```python
from build123d import *

# Parameters (mm, degrees)
EXTRUDE_THIN2_OUTLINE_R   = 5.5
EXTRUDE_THIN2_OUTLINE_R_2 = 3.5
EXTRUDE_THIN2_DEPTH       = 45
EXTRUDE_THIN2_2_OUTLINE_R = 3.5
EXTRUDE_THIN2_2_DEPTH     = 2
EXTRUDE_THIN2_START       = 43
EXTRUDE_THIN2_3_OUTLINE_R = 3.5
EXTRUDE_THIN2_3_DEPTH     = 2
EXTRUDE_THIN2_4_DEPTH     = 45
EXTRUDE_THIN2_5_DEPTH     = 45
EXTRUDE_THIN2_6_DEPTH     = 45
EXTRUDE_THIN2_7_DEPTH     = 45
EXTRUDE_THIN2_8_OUTLINE_W = 2
EXTRUDE_THIN2_8_OUTLINE_H = 52
EXTRUDE_THIN2_8_DEPTH     = 45
SKETCH4_R                 = 5.5
BOSS_EXTRUDE2_DEPTH       = 0.001
SKETCH6_R                 = 6.759527971
BOSS_EXTRUDE3_DEPTH       = 1
SCALE1_SCALE              = 1.5


# Read off the part's stored shape, not the designer's step: Extrude-Thin2
with BuildPart() as part:
    # Extrude-Thin2 outline → Extrude-Thin2 (new body)
    with BuildSketch(Plane(origin=(0, 0, 0), x_dir=(1, 0, 0), z_dir=(0, 1, 0))):
        Circle(EXTRUDE_THIN2_OUTLINE_R)
        Circle(EXTRUDE_THIN2_OUTLINE_R_2, mode=Mode.SUBTRACT)
    extrude(amount=EXTRUDE_THIN2_DEPTH)

    # Extrude-Thin2 2 outline → Extrude-Thin2 2 (add)
    with BuildSketch(Plane(origin=(0, 0, 0), x_dir=(1, 0, 0), z_dir=(0, 1, 0))):
        Circle(EXTRUDE_THIN2_2_OUTLINE_R)
    extrude(amount=EXTRUDE_THIN2_2_DEPTH)

    # Extrude-Thin2 3 outline → Extrude-Thin2 3 (add)
    with BuildSketch(Plane(origin=(0, 0, 0), x_dir=(1, 0, 0), z_dir=(0, 1, 0)).offset(EXTRUDE_THIN2_START)):
        Circle(EXTRUDE_THIN2_3_OUTLINE_R)
    extrude(amount=EXTRUDE_THIN2_3_DEPTH)



with BuildPart() as body_2:
    # Extrude-Thin2 4 outline → Extrude-Thin2 4 (new body)
    with BuildSketch(Plane(origin=(0, 0, 0), x_dir=(1, 0, 0), z_dir=(0, 1, 0))):
        Polygon((-3.970737329, 2.341632991), (-53.425676176, 18.410516698), (-54.043710165, 16.508403666), (-4.588771318, 0.439519958), align=None)
    extrude(amount=EXTRUDE_THIN2_4_DEPTH)


with BuildPart() as body_3:
    # Extrude-Thin2 5 outline → Extrude-Thin2 5 (new body)
    with BuildSketch(Plane(origin=(0, 0, 0), x_dir=(1, 0, 0), z_dir=(0, 1, 0))):
        Polygon((-3.45405063, -3.052791222), (-34.018883749, -45.12167493), (-32.40084976, -46.297245434), (-1.836016641, -4.228361727), align=None)
    extrude(amount=EXTRUDE_THIN2_5_DEPTH)


with BuildPart() as body_4:
    # Extrude-Thin2 6 outline → Extrude-Thin2 6 (new body)
    with BuildSketch(Plane(origin=(0, 0, 0), x_dir=(1, 0, 0), z_dir=(0, 1, 0))):
        Polygon((1.836016641, -4.228361727), (32.40084976, -46.297245434), (34.018883749, -45.12167493), (3.45405063, -3.052791222), align=None)
    extrude(amount=EXTRUDE_THIN2_6_DEPTH)


with BuildPart() as body_5:
    # Extrude-Thin2 7 outline → Extrude-Thin2 7 (new body)
    with BuildSketch(Plane(origin=(0, 0, 0), x_dir=(1, 0, 0), z_dir=(0, 1, 0))):
        Polygon((4.588771318, 0.439519958), (54.043710165, 16.508403666), (53.425676176, 18.410516698), (3.970737329, 2.341632991), align=None)
    extrude(amount=EXTRUDE_THIN2_7_DEPTH)


with BuildPart() as body_6:
    # Extrude-Thin2 8 outline → Extrude-Thin2 8 (new body)
    with BuildSketch(Plane(origin=(0, 0, 0), x_dir=(1, 0, 0), z_dir=(0, 1, 0))):
        with Locations((0, 30.5)):
            Rectangle(EXTRUDE_THIN2_8_OUTLINE_W, EXTRUDE_THIN2_8_OUTLINE_H)
    extrude(amount=EXTRUDE_THIN2_8_DEPTH)


with BuildPart() as part_1:
    add(part.part)

    add(body_2.part)  # Boss-Extrude2 merges body 2

    add(body_3.part)  # Boss-Extrude2 merges body 3

    add(body_4.part)  # Boss-Extrude2 merges body 4

    add(body_5.part)  # Boss-Extrude2 merges body 5

    add(body_6.part)  # Boss-Extrude2 merges body 6
    # Sketch4 → Boss-Extrude2 (add)
    with BuildSketch(Plane(origin=(0, 45, 0), x_dir=(1, 0, 0), z_dir=(0, 1, 0))):
        with Locations(Location((0, 0, 0), (0, 0, 79.524318304))):
            Circle(SKETCH4_R)
    extrude(amount=BOSS_EXTRUDE2_DEPTH)

    # Sketch6 → Boss-Extrude3 (add)
    with BuildSketch(Plane(origin=(0, 45, 0), x_dir=(1, 0, 0), z_dir=(0, 1, 0))):
        with Locations(Location((0, 0, 0), (0, 0, 81.492473787))):
            Circle(SKETCH6_R)
    extrude(amount=BOSS_EXTRUDE3_DEPTH)


with BuildPart() as part_2:
    # Scale1: scaled about (0, 22.627935727, 1e-09)
    add(part_1.part.scale(SCALE1_SCALE).moved(Location((0, -11.313967864, -1e-09))))


solid = part_2.part
```
The model under review builds one solid part; all positions refer to its coordinate system, in mm. A direction names the side the tool comes from. Coordinates: 2 decimals unless noted, no trailing zeros. Write each loop counter-clockwise with the first axis right and the second up, starting at its lowest first coordinate (ties: lowest second). Pieces come first, ordered by that corner, then holes. Notation, with made-up numbers: (1, 40.5) - (31, 40.5) arc R23 cw to (31, 75.5) - close; hole circle Ø3 at (53, 70.25). An arc over 180 degrees is marked (long way). Answer in a Markdown table with one row per item. Add a question column.
Q1. Draft analysis for pull direction Y (two halves, no side actions). For faces 5 (the face through (-1.138, 22.006, 5.125)), 6 (the face through (8, 56.186, 3)), 7 (the face through (45, 56.186, -15)), state which applies: +Y half, -Y half, draft (parallel to the pull), parting line (faces both ways), or undercut.
Q2. Clearance check with flat-ended pins moving along their axes: pin 1 (23 mm diameter, centred on x = 31.5, z = 38, fed in from +Y); pin 2 (2 mm diameter, centred on y = 21.5, z = 1.5, fed in from -X); pin 3 (1.3 mm diameter, centred on x = -0.5, z = 9, fed in from -Y). State where each tip first meets the part, or that it passes through.
Q3. Consider section A-A on y = -2. Give the boundary of the cut face in (x, z), then the cut area to 3 significant figures.
Q4. Consider section D-D on x = -60. Give the boundary of the cut face in (y, z).
Q5. Consider section B-B on z = 30. Give the boundary of the cut face in (x, y).
Q6. Consider section C-C on x = 22.5. Give the boundary of the cut face in (y, z), then the cut area to 3 significant figures.
Q7. For faces 1 (the face through (0, -8.314, 0)), 2 (the face through (7.83, 21.96, 2.6)), 3 (the face through (-0.05, 21.96, 8.25)), 4 (the face through (9.464, 56.926, 3.638)), list the 3-axis set-ups (+Z, -Z, +X, -X, +Y, -Y) from which the entire face can be reached by the end or side of a thin tool; tool diameter is ignored.
Q8. To check wall thickness, follow line 1 along X through (y, z) = (28.5, 0); line 2 along Y through (x, z) = (0.5, 0); line 3 along X through (y, z) = (17.5, -47.5). State the ranges of each line that lie inside material, in increasing order. Write a range as from..to.
Answers below:
| question | item | result |
|---|---|---|
| 1 | face 5 | undercut |
| 1 | face 6 | -Y half |
| 1 | face 7 | +Y half |
| 2 | pin 1 | y = 56.19 |
| 2 | pin 2 | x = -8.23 |
| 2 | pin 3 | y = 56.19 |
| 3 | outline | (-81.07, -24.76) - (-80.14, -27.62) - (-7.25, -3.93) arc R8.25 ccw to (-1.5, -8.11) - (-1.5, -84.75) - (1.5, -84.75) - (1.5, -8.11) arc R8.25 ccw to (7.25, -3.93) - (80.14, -27.62) - (81.07, -24.76) - (8.18, -1.08) arc R8.25 ccw to (5.98, 5.68) - (51.03, 67.68) - (48.6, 69.45) - (3.55, 7.44) arc R8.25 ccw to (-3.55, 7.44) - (-48.6, 69.45) - (-51.03, 67.68) - (-5.98, 5.68) arc R8.25 ccw to (-8.18, -1.08) - close; hole circle Ø10.5 at (0, 0) |
| 3 | area | 1,280 mm² |
| 4 | outline | (-11.31, -21.07) - (56.19, -21.07) - (56.19, -17.92) - (-11.31, -17.92) - close |
| 5 | outline | (-23.65, -11.31) - (-19.94, -11.31) - (-19.94, 56.19) - (-23.65, 56.19) - close; (19.94, -11.31) - (23.65, -11.31) - (23.65, 56.19) - (19.94, 56.19) - close |
| 6 | outline | (-11.31, -8.89) - (56.19, -8.89) - (56.19, -5.73) - (-11.31, -5.73) - close; (-11.31, 28.42) - (56.19, 28.42) - (56.19, 33.52) - (-11.31, 33.52) - close |
| 6 | area | 557 mm² |
| 7 | face 1 | none |
| 7 | face 2 | +X, -Y |
| 7 | face 3 | +Z, -Y |
| 7 | face 4 | +Y |
| 8 | line 1 | -8.25..-5.25, 5.25..8.25 |
| 8 | line 2 | -11.31..-8.31, 53.19..57.69 |
| 8 | line 3 | -1.5..1.5 |
